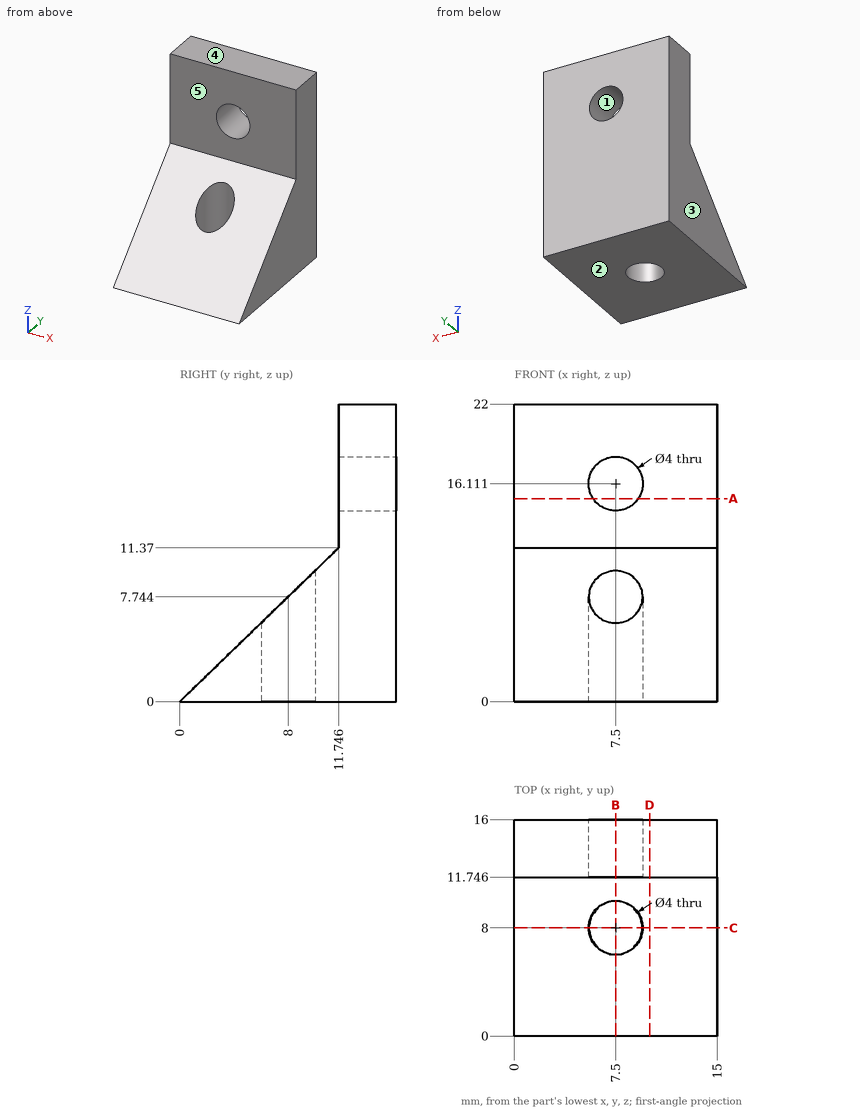
Can you work these out from the drawing? Everything is in mm from the part's minimum corner. A direction names the side the tool comes from. Give positions to 0.01 mm unless a question says otherwise; leave off trailing zeros. Loops run counter-clockwise (first coordinate to the right, second up) from the corner with the lowest first, then second, coordinate; pieces in that order, holes last. Notation, with made-up numbers: (62.5, -32) -> (114.5, -32) arc R17 cw to (114.5, -21) -> close; hole circle Ø11 at (17.5, -28). An arc over 180 degrees is marked (long way). Return JSON: item names as keys, results as strings.
Item 1: We'd pull the mould along X, two halves only. Please class the marked faces 1, 2 and 3: +X half, -X half, draft (parallel to the pull), parting line (faces both ways), or undercut.
Geometry results:
{"face 1": "undercut", "face 2": "draft", "face 3": "-X half"}
Item 2: I'm going to push flat-ended pins straight in: pin 1 (3 mm diameter, centred on x = 6.5, z = 15.5, fed in from -Y); pin 2 (4.5 mm diameter, centred on x = 7.5, y = 8, fed in from +Z). Where does each tip first touch, or does it pass through?
Geometry results:
{"pin 1": "stops at y = 11.75", "pin 2": "stops at z = 9.92"}
Item 3: I need wall thicknesses on L1, parallel to Z at x = 7.5, y = 13.8; L2, parallel to X at y = 8, z = 4; L3, parallel to Y at x = 12.25, z = 12.25. Which ranges of each line are inside material? Lowest first, please. Write a range as from..to.
Geometry results:
{"L1": "z = 0..14.11, 18.11..22", "L2": "x = 0..5.5, 9.5..15", "L3": "y = 11.75..16"}
Item 4: Which directions (+Z, -Z, +X, -X, +Y, -Y) give clear straight access to the entire face, cutting with the end or side of a thin tool? Please do the marked faces 4 and 5.
Geometry results:
{"face 4": "+Z, +X, -X, +Y, -Y", "face 5": "+Z, +X, -X, -Y"}
Item 5: If we section it at D-D on x = 10: List the corners of the cut face in (y, z) for me.
Geometry results:
{"outline": "(0, 0) -> (16, 0) -> (16, 22) -> (11.75, 22) -> (11.75, 11.37) -> close"}
Item 6: If we section it at C-C on y = 8: List the corners of the cut face in (x, z) for me, plus the area to 3 significant figures.
Geometry results:
{"outline": "(0, 0) -> (5.5, 0) -> (5.5, 7.74) -> (0, 7.74) -> close; (9.5, 0) -> (15, 0) -> (15, 7.74) -> (9.5, 7.74) -> close", "area": "85.2 mm²"}
Item 7: If we section it at B-B on x = 7.5: List the corners of the cut face in (y, z) for me, plus the area to 3 significant figures.
Geometry results:
{"outline": "(0, 0) -> (6, 0) -> (6, 5.81) -> close; (10, 0) -> (16, 0) -> (16, 14.11) -> (11.75, 14.11) -> (11.75, 11.37) -> (10, 9.68) -> close; (11.75, 18.11) -> (16, 18.11) -> (16, 22) -> (11.75, 22) -> close", "area": "112 mm²"}
Item 8: If we section it at A-A on z = 15: List the corners of the cut face in (x, y) for me.
Geometry results:
{"outline": "(0, 11.75) -> (5.84, 11.75) -> (5.84, 16) -> (0, 16) -> close; (9.16, 11.75) -> (15, 11.75) -> (15, 16) -> (9.16, 16) -> close"}
